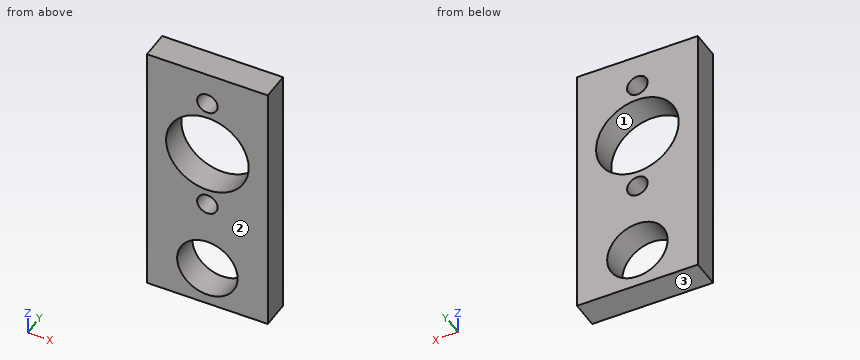
Solid Edge part; units mm, degrees
sketch "Sketch1" plane through (0, 0, 0) normal (0, -1, 0) x (1, 0, 0)
  line L0 (60, 0) -> (60, 130)
  line L1 (60, 130) -> (0, 130)
  line L2 (0, 130) -> (0, 57.7585)
  line L3 (0, 57.7585) -> (0, 0)
  line L4 (0, 0) -> (60, 0)
extrude "Protrusion1" add sketch "Sketch1" along normal blind 14.1635
sketch "Sketch2" plane through (0, 0, 0) normal (0, -1, 0) x (1, 0, 0)
  circle A0 centre (30, 113.6) radius 5.1
  circle A1 centre (30, 85) radius 20.5
  circle A2 centre (30, 56.4) radius 5.1
  circle A3 centre (30, 20) radius 15
extrude "ExtrudedCutout_1" cut sketch "Sketch2" along normal blind 65.8643
Check sheet for the modelled part. Datum: model origin and axes. Units: mm. Face numbers are marked on the shaded views. Round coordinates to 2 decimals unless told otherwise and drop trailing zeros. Order: outer loops, then holes, each group sorted by start corner. A loop starts at its lowest first (then second) coordinate and runs counter-clockwise, first axis right, second up.
Q1. Scan lines: L1, parallel to Z at x = 30, y = -7.75; L2, parallel to X at y = -4.75, z = 85; L3, parallel to Z at x = 31, y = -7. Record each from-to range of solid material in increasing order.
Filled sheet:
L1: z = 0 to 5, 35 to 51.3, 61.5 to 64.5, 105.5 to 108.5, 118.7 to 130
L2: x = 0 to 9.5, 50.5 to 60
L3: z = 0 to 5.03, 34.97 to 51.4, 61.4 to 64.52, 105.48 to 108.6, 118.6 to 130
Q2. Cross-section at C-C, the plane y = -9.75. Enter the section's corners in (x, z), plus the area to 3 significant figures.
Filled sheet:
outline: (0, 0) - (60, 0) - (60, 130) - (0, 130) - close; hole circle Ø41 at (30, 85); hole circle Ø30 at (30, 20); hole circle Ø10.2 at (30, 56.4); hole circle Ø10.2 at (30, 113.6)
area: 5,610 mm2
Q3. Cross-section at A-A, the plane z = 20. Enter the section's corners in (x, y), plus the area to 3 significant figures.
Filled sheet:
outline: (0, -14.16) - (15, -14.16) - (15, 0) - (0, 0) - close; (45, -14.16) - (60, -14.16) - (60, 0) - (45, 0) - close
area: 425 mm2
Q4. Cross-section at B-B, the plane x = 30. Enter the section's corners in (y, z), plus the area to 3 significant figures.
Filled sheet:
outline: (-14.16, 0) - (0, 0) - (0, 5) - (-14.16, 5) - close; (-14.16, 35) - (0, 35) - (0, 51.3) - (-14.16, 51.3) - close; (-14.16, 61.5) - (0, 61.5) - (0, 64.5) - (-14.16, 64.5) - close; (-14.16, 105.5) - (0, 105.5) - (0, 108.5) - (-14.16, 108.5) - close; (-14.16, 118.7) - (0, 118.7) - (0, 130) - (-14.16, 130) - close
area: 547 mm2
Q5. Draft check along Z on the marked faces 1, 2 and 3. Enter one of: pulls with the +Z half, pulls with the -Z half, needs draft (parallel to the pull), parting line crosses it, or undercut.
Filled sheet:
face 1: undercut
face 2: needs draft
face 3: pulls with the -Z half
Q6. Cross-section at D-D, the plane z = 89.5. Enter the section's corners in (x, y).
Filled sheet:
outline: (0, -14.16) - (10, -14.16) - (10, 0) - (0, 0) - close; (50, -14.16) - (60, -14.16) - (60, 0) - (50, 0) - close
